Input: dimensioned drawing with shaded views. Units: mm. Origin: part minimum x, y, z. A direction names the side the tool comes from. Coordinates: 2 decimals unless noted, no trailing zeros. Order: outer loops, then holes, each group sorted by start corner. A loop starts at its lowest first (then second) coordinate and runs counter-clockwise, first axis right, second up. Notation, with made-up numbers: (-1.75, 28.25) -> (52.25, 28.25) arc R15 cw to (52.25, 42.25) -> close; hole circle Ø6 at (15, 16). An arc over 180 degrees is marked (long way). Put each result on its own line as item: value.
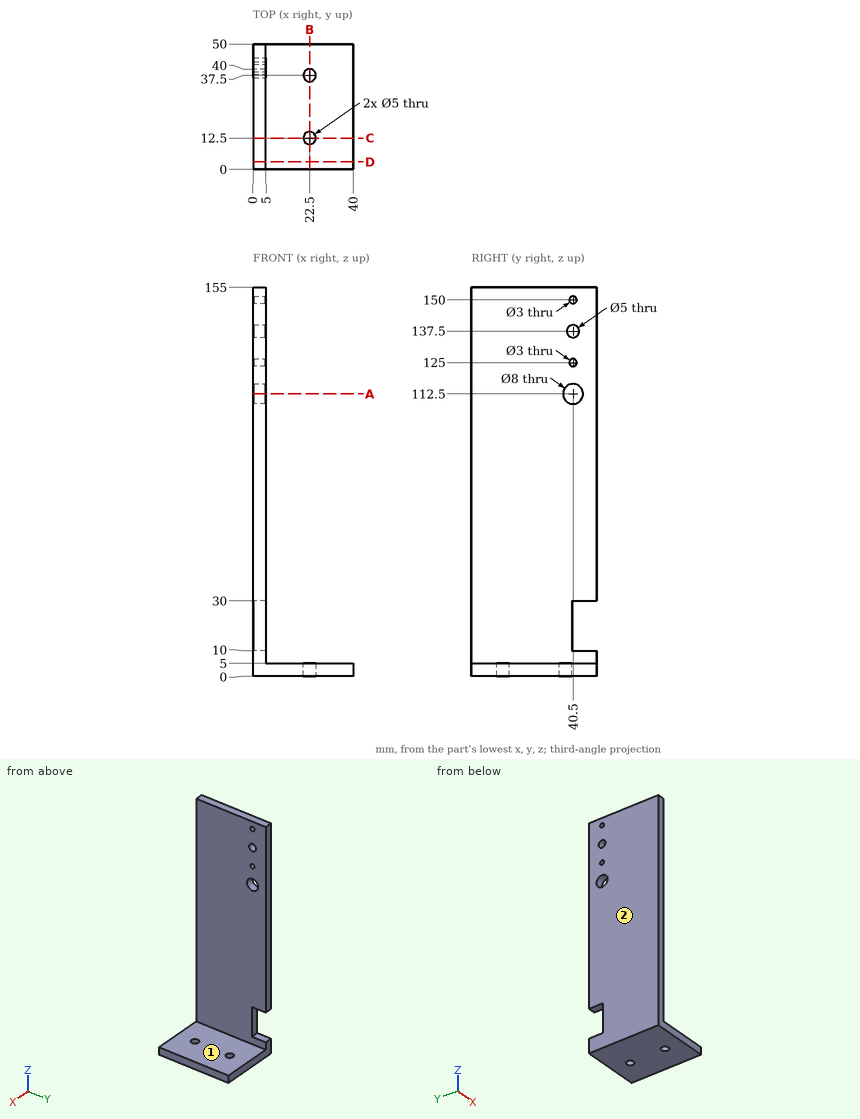
1. Set-up query: the marked faces 1 and 2. Return all of +Z, -Z, +X, -X, +Y, -Y with unobstructed straight access to the full face (end or side cutting, diameter ignored); none if empty.
Numbers:
face 1: +Z, +X, +Y, -Y
face 2: +Z, -Z, -X, +Y, -Y
2. Ray query, line 1 along Y through (x, z) = (22, 2); line 2 along Y through (x, z) = (3, 112); line 3 along X through (y, z) = (7, 138). Return the intervals inside material, ascending.
Numbers:
line 1: y = 0 to 10.05, 14.95 to 35.05, 39.95 to 50
line 2: y = 0 to 36.53, 44.47 to 50
line 3: x = 0 to 5
3. Cut plane C-C on y = 12.5. Output: boundary loops of the cut face in (x, z), plus the area to 3 significant figures.
Numbers:
outline: (0, 0) -> (20, 0) -> (20, 5) -> (5, 5) -> (5, 155) -> (0, 155) -> close; (25, 0) -> (40, 0) -> (40, 5) -> (25, 5) -> close
area: 925 mm2
4. Cut plane A-A on z = 112.5. Output: boundary loops of the cut face in (x, y), plus the area to 3 significant figures.
Numbers:
outline: (0, 0) -> (5, 0) -> (5, 36.5) -> (0, 36.5) -> close; (0, 44.5) -> (5, 44.5) -> (5, 50) -> (0, 50) -> close
area: 210 mm2
5. Cut plane D-D on y = 3. Output: boundary loops of the cut face in (x, z).
Numbers:
outline: (0, 0) -> (40, 0) -> (40, 5) -> (5, 5) -> (5, 155) -> (0, 155) -> close
6. First-contact query: pin 1 (1.5 mm diameter, centred on x = 1.5, z = 19.5, fed in from +Y); pin 2 (15 mm diameter, centred on y = 35, z = 86, fed in from +X); pin 3 (10.5 mm diameter, centred on x = 28, y = 19.5, fed in from +Z). Flat tips, straight axial feed; report the tip coordinate or a pass-through.
Numbers:
pin 1: stops at y = 40
pin 2: stops at x = 5
pin 3: stops at z = 5
7. Cut plane B-B on x = 22.5. Output: boundary loops of the cut face in (y, z).
Numbers:
outline: (0, 0) -> (10, 0) -> (10, 5) -> (0, 5) -> close; (15, 0) -> (35, 0) -> (35, 5) -> (15, 5) -> close; (40, 0) -> (50, 0) -> (50, 5) -> (40, 5) -> close
